from build123d import *

# Parameters (mm, degrees)
CROQUIS1_W              = 6
CROQUIS1_H              = 10
SALIENTE_EXTRUIR1_DEPTH = 6
CROQUIS2_W              = 4
CROQUIS2_H              = 7
SALIENTE_EXTRUIR3_DEPTH = 4
CROQUIS4_W              = 4
CROQUIS4_H              = 4
CORTAR_EXTRUIR1_DEPTH   = 2
SALIENTE_EXTRUIR5_DEPTH = 4


with BuildPart() as part:
    # Croquis1 → Saliente-Extruir1 (new body)
    with BuildSketch(Plane(origin=(0, 0, 0), x_dir=(1, 0, 0), z_dir=(0, 1, 0))):
        Rectangle(CROQUIS1_W, CROQUIS1_H)
    extrude(amount=SALIENTE_EXTRUIR1_DEPTH)

    # Croquis2 → Saliente-Extruir3 (add)
    with BuildSketch(Plane(origin=(0, 6, 0), x_dir=(1, 0, 0), z_dir=(0, 1, 0))):
        with Locations((-1, 0.012360782)):
            Rectangle(CROQUIS2_W, CROQUIS2_H)
    extrude(amount=SALIENTE_EXTRUIR3_DEPTH)

    # Croquis4 → Cortar-Extruir1 (cut)
    with BuildSketch(Plane(origin=(0, 10, 0), x_dir=(1, 0, 0), z_dir=(0, 1, 0))):
        with Locations((-1, 0.012360782)):
            Rectangle(CROQUIS4_W, CROQUIS4_H)
    extrude(amount=-CORTAR_EXTRUIR1_DEPTH, mode=Mode.SUBTRACT)

    # Croquis6 → Saliente-Extruir5 (add)
    with BuildSketch(Plane.XY.offset(-2.012360782)):
        Polygon((-3, 10), (1, 8), (-3, 8), align=None)
    extrude(amount=SALIENTE_EXTRUIR5_DEPTH)


solid = part.part
Here's how the part is built. I have some questions about the finished solid (model axes, mm). A direction names the side the tool comes from. Coordinates: 2 decimals unless noted, no trailing zeros. Loops run counter-clockwise (first coordinate to the right, second up) from the corner with the lowest first, then second, coordinate; pieces in that order, holes last.
1. For P1, Ø1.6, axis at x = -1, y = 8.5, coming from the -Z side; P2, Ø0.6, axis at x = 0, y = 9, coming from the +Z side, each with a flat end and sliding along its axis, tell me the tip position at first contact or that it passes through.
2. For faces 4 (the flat face through (1, 7.5, 0)), 5 (the flat face through (0, 9, -2.012)), 6 (the flat face through (-1, 8, -3.512)), 7 (the flat face through (-3, 5, 0)), which set-ups out of +Z, -Z, +X, -X, +Y, -Y let a thin tool reach every point of the face, with its end or its side?
3. Imagine slicing it at C-C, the plane y = 8.25. Please give me the cut outline in (x, z), and give its area (3 significant figures).
4. Imagine slicing it at B-B, the plane z = -1.5. Please give me the cut outline in (x, y), and give its area (3 significant figures).
5. Imagine slicing it at D-D, the plane x = 0.6. Please give me the cut outline in (y, z).
6. Imagine slicing it at A-A, the plane x = -0.4. Please give me the cut outline in (y, z).
7. I need wall thicknesses on L1, parallel to Y at x = 2.6, z = -1.25; L2, parallel to X at y = 7.5, z = -2.5; L3, parallel to Z at x = 0.35, y = 7.5. Which ranges of each line are inside material? Lowest first, please.
8. If we mould it in two halves opening along Y, with no side actions, what happens to faces 1 (the flat face through (-1, 9, 0)), 2 (the flat face through (0, 0, 0)), 3 (the flat face through (-1, 8, 3.488))? For each: pulls with the +Y half, pulls with the -Y half, needs draft (parallel to the pull), parting line crosses it, or undercut.
Taken from the geometry:
1. P1: stops at z = -3.51
1. P2: stops at z = 3.49
2. face 4: +Z, -Z, +X, +Y
2. face 5: +X, +Y
2. face 6: -Z, +X, -X, +Y
2. face 7: +Z, -Z, -X, +Y, -Y
3. outline: (-3, -3.51) - (1, -3.51) - (1, -2.01) - (0.5, -2.01) - (0.5, 1.99) - (1, 1.99) - (1, 3.49) - (-3, 3.49) - close
3. area: 26.0 mm2
4. outline: (-3, 0) - (3, 0) - (3, 6) - (1, 6) - (1, 8) - (-3, 10) - close
4. area: 48.0 mm2
5. outline: (0, -5) - (6, -5) - (6, -3.51) - (10, -3.51) - (10, -2.01) - (8.2, -2.01) - (8.2, 1.99) - (10, 1.99) - (10, 3.49) - (6, 3.49) - (6, 5) - (0, 5) - close
6. outline: (0, -5) - (6, -5) - (6, -3.51) - (10, -3.51) - (10, -2.01) - (8.7, -2.01) - (8.7, 1.99) - (10, 1.99) - (10, 3.49) - (6, 3.49) - (6, 5) - (0, 5) - close
7. L1: y = 0 to 6
7. L2: x = -3 to 1
7. L3: z = -3.51 to 3.49
8. face 1: pulls with the +Y half
8. face 2: pulls with the -Y half
8. face 3: needs draft
